Autodesk Inventor part; units mm, degrees
ref_plane "YZ Plane" through (0, 0, 0) normal (1, 0, 0) x (0, 1, 0)
ref_plane "XZ Plane" through (0, 0, 0) normal (0, 1, 0) x (-1, 0, 0)
ref_plane "XY Plane" through (0, 0, 0) normal (0, 0, 1) x (1, 0, 0)
sketch "Sketch1" plane through (0, 0, 0) normal (0, 0, 1) x (1, 0, 0)
  circle A0 centre (0, 0) radius 100
  line L0 (-117.4264, -75) -> (-117.4264, 75)
  line L1 (-117.4264, 75) -> (-75, 117.4264)
  line L2 (-75, 117.4264) -> (75, 117.4264)
  line L3 (75, 117.4264) -> (117.4264, 75)
  line L4 (117.4264, 75) -> (117.4264, -75)
  line L5 (117.4264, -75) -> (75, -117.4264)
  line L6 (75, -117.4264) -> (-75, -117.4264)
  line L7 (-75, -117.4264) -> (-117.4264, -75)
  point P0 (-117.4264, 0)
  point P1 (117.4264, 0)
  point P2 (0, 117.4264)
  point P3 (0, -117.4264)
  dimension "d22" = 200
  dimension "d33" = 150
  dimension "d35" = 60
extrude "Plate1" add sketch "Sketch1" along normal blind 3
equation "\"d33\" = Wall_1_width"
equation "\"d35\" = Wall_2_width"
equation "\"d2\" = Thickness"
equation "\"BendReliefWidth\" = Thickness"
equation "\"BendReliefDepth\" = 0.5 * Thickness"
equation "\"CornerReliefSize\" = 4 * Thickness"
equation "\"MinimumRemnant\" = 2 * Thickness"
equation "\"TransitionRadius\" = BendRadius"
equation "\"JacobiRadiusSize\" = BendRadius"
equation "\"GapSize\" = Thickness"
equation "\"Wall_1_width\" = 150"
equation "\"Wall_2_width\" = 60"
properties part number "TKS 3553 BOTTOM DS reduce flange" material "Stainless Steel"
Input: part model. Units: mm. Frame: model coordinates. Give positions to 0.01 mm unless a question says otherwise; leave off trailing zeros. Write each loop counter-clockwise with the first axis right and the second up, starting at its lowest first coordinate (ties: lowest second). Pieces come first, ordered by that corner, then holes.
Q1. Section A-A, the plane x = 0. Output: boundary loops of the cut face in (y, z), plus the area to 3 significant figures.
Q2. Material intervals for probe 1 along Y at (x, z) = (0, 1.6); probe 2 along X at (y, z) = (5, 1.75); probe 3 along X at (y, z) = (-89, 2.65), sorted ascending.
Q3. Section B-B, the plane z = 1.2. Output: boundary loops of the cut face in (x, y).
Q4. Pull-direction query (Y, two-part tool) for faces 1 (the face through (96.51, -95.916, 1.479)), 2 (the face through (-106, 2, 3)), 3 (the face through (95.916, 96.51, 1.479)), 4 (the face through (95.38, -30.04, 1.48)); classes: pulls with the +Y half, pulls with the -Y half, needs draft (parallel to the pull), parting line crosses it, or undercut.
Filled in:
1. outline: (-117.43, 0) - (-100, 0) - (-100, 3) - (-117.43, 3) - close; (100, 0) - (117.43, 0) - (117.43, 3) - (100, 3) - close
1. area: 105 mm2
2. probe 1: y = -117.43 to -100, 100 to 117.43
2. probe 2: x = -117.43 to -99.87, 99.87 to 117.43
2. probe 3: x = -103.43 to -45.6, 45.6 to 103.43
3. outline: (-117.43, -75) - (-75, -117.43) - (75, -117.43) - (117.43, -75) - (117.43, 75) - (75, 117.43) - (-75, 117.43) - (-117.43, 75) - close; hole circle Ø200 at (0, 0)
4. face 1: pulls with the -Y half
4. face 2: needs draft
4. face 3: pulls with the +Y half
4. face 4: undercut
